Autodesk Inventor part; units mm, degrees
ref_plane "YZ Plane" through (0, 0, 0) normal (1, 0, 0) x (0, 1, 0)
ref_plane "XZ Plane" through (0, 0, 0) normal (0, 1, 0) x (-1, 0, 0)
ref_plane "XY Plane" through (0, 0, 0) normal (0, 0, 1) x (1, 0, 0)
sketch "Sketch1" plane through (0, 0, 0) normal (1, 0, 0) x (0, 1, 0)
  line L0 (13.7403, 22.0625) -> (-11.6597, 22.0625)
  line L1 (-11.6597, 22.0625) -> (-11.6597, -3.3375)
  line L2 (-11.6597, -3.3375) -> (13.7403, -3.3375)
  line L3 (13.7403, -3.3375) -> (13.7403, 22.0625)
  point P0 (0, 0)
  dimension "d0" = 25.4
  dimension "d1" = 25.4
extrude "Extrusion1" add sketch "Sketch1" along normal blind 101.6
sketch "Sketch2" plane through (0, 13.7403, 22.0625) normal (0, 1, 0) x (1, 0, 0)
  circle A0 centre (50.8, 12.7) radius 7.5047
  line L0 (0, 25.4) -> (0, 0)
  line L1 (0, 25.4) -> (101.6, 25.4)
  point P0 (0, 22.0625)
  dimension "d4" = 50.8
  dimension "d5" = 12.7
extrude "Extrusion2" cut sketch "Sketch2" against normal blind 101.6
properties part number "ServoBlock"
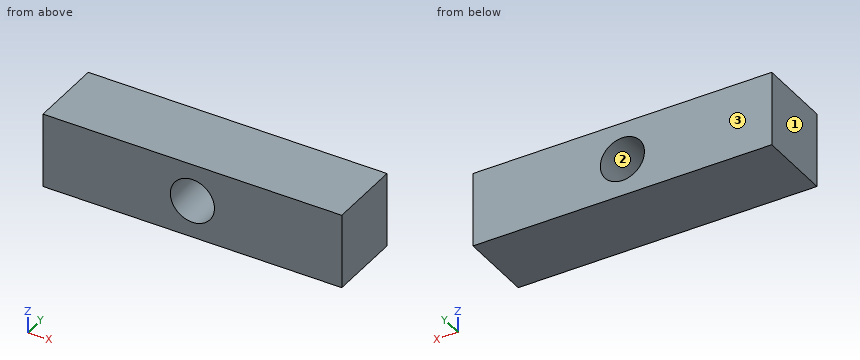
Could you check a few things on this model? Use its own coordinates, in mm. Face numbers are marked on the shaded views. Give positions to 0.01 mm unless a question says otherwise; leave off trailing zeros. Loops run counter-clockwise (first coordinate to the right, second up) from the corner with the lowest first, then second, coordinate; pieces in that order, holes last. Notation, with made-up numbers: (43, 9) -> (51, 9) arc R8 ccw to (51, 21) -> close; hole circle Ø7 at (27.5, 70.5). An arc over 180 degrees is marked (long way). Put each result on its own line as item: value.
(1) Thinking about a two-plate mould opening in X: for the marked faces 1, 2 and 3, which applies, pulls with the +X half, pulls with the -X half, needs draft (parallel to the pull), parting line crosses it, or undercut?
Computed:
face 1: pulls with the -X half
face 2: undercut
face 3: needs draft
(2) Imagine slicing it at C-C on y = 12. Write out the boundary of the cut face in (x, z), plus the area to 3 significant figures.
Computed:
outline: (0, -3.34) -> (101.6, -3.34) -> (101.6, 22.06) -> (0, 22.06) -> close; hole circle Ø15.01 at (50.8, 9.36)
area: 2,400 mm^2
(3) Imagine slicing it at B-B on z = 4.5. Write out the boundary of the cut face in (x, y).
Computed:
outline: (0, -11.66) -> (45.08, -11.66) -> (45.08, 13.74) -> (0, 13.74) -> close; (56.52, -11.66) -> (101.6, -11.66) -> (101.6, 13.74) -> (56.52, 13.74) -> close
(4) Please list where these lines run through material, in increasing order: probe 1 along Z at (x, y) = (50.8, -1.5); probe 2 along X at (y, z) = (11, 9.5); probe 3 along X at (y, z) = (-9.25, 14.25). Write a range as [from, to].
Computed:
probe 1: [-3.34, 1.86], [16.87, 22.06]
probe 2: [0, 43.3], [58.3, 101.6]
probe 3: [0, 45.11], [56.49, 101.6]
(5) Imagine slicing it at A-A on x = 51.5. Write out the boundary of the cut face in (y, z), plus the area to 3 significant figures.
Computed:
outline: (-11.66, -3.34) -> (13.74, -3.34) -> (13.74, 1.89) -> (-11.66, 1.89) -> close; (-11.66, 16.83) -> (13.74, 16.83) -> (13.74, 22.06) -> (-11.66, 22.06) -> close
area: 266 mm^2
(6) I'm going to push a flat-ended pin straight in: pin 1 Ø4 at (y, z) = (3, 7) entering from -X. Where does the tip first touch, or does it pass through?
Computed:
pin 1: x = 0
